CAD build for the part. Positions are in the model's coordinates, mm. Round coordinates to 2 decimals unless told otherwise and drop trailing zeros. Loops run counter-clockwise (first coordinate to the right, second up) from the corner with the lowest first, then second, coordinate; pieces in that order, holes last. Notation, with made-up numbers: M 53,26 L 87,26 A7 cw 87,33 Z; hole C 78.5,10 d8. An arc over 180 degrees is marked long. Use one line per item in the form item = value.
from build123d import *

# Parameters (mm, degrees)
F2_W     = 25.146
F2_H     = 4.7498
F3_DEPTH = 34.6974
F4_R     = 0.381


with BuildPart() as f1:
    # F0 (on Right) → F1 (revolve)
    with BuildSketch(Plane.YZ):
        Polygon((-12.6492, 0.1524), (-12.6492, 34.6964), (-16.6624, 34.6964), (-16.6624, 31.6484), (-13.8938, 31.6484), (-13.8938, 12.8524), (-13.2842, 0.1524), align=None)
    revolve(axis=Axis((0, 0, 4.6482), (0, 0, -1)))

    # F2 (on Top) → F3 (cut, through all)
    with BuildSketch(Plane.XY):
        with Locations((-12.827, 0)):
            Rectangle(F2_W, F2_H)
    extrude(amount=F3_DEPTH, mode=Mode.SUBTRACT)

    # F4
    f4_edges = [f1.edges().sort_by_distance(p)[0] for p in [
        (-13.379864, -2.3749, 6.502395),
        (-13.689322, -2.3749, 22.2504),
        (-13.379864, 2.3749, 6.502395),
        (-13.689322, 2.3749, 22.2504),
        (-15.090803, -2.3749, 31.6484),
        (-15.090803, 2.3749, 31.6484),
        (12.6492, 0, 34.6964),
        (13.8938, 0, 12.8524),
    ]]
    fillet(f4_edges, radius=F4_R)


solid = f1.part
1. Probe line 1 along Y through (x, z) = (0, 15); line 2 along Y through (x, z) = (3.5, 6); line 3 along X through (y, z) = (10.5, 4). List the from-to ranges inside material, lowest first. Write a range as from..to.
Completed:
line_1 = -13.89..-12.65, 12.65..13.89
line_2 = -13.11..-12.16, 12.16..13.11
line_3 = -8.44..-7.05, 7.05..8.44
2. Cut at C-C on z = 13.5. Write the cut outline in (x, y), and give its area (3 significant figures).
Completed:
outline = M -13.6,-2.83 A13.89 ccw long -13.6,2.83 A0.38 ccw -13.23,2.37 L -12.42,2.37 A12.65 cw long -12.42,-2.37 L -13.23,-2.37 A0.38 ccw Z
area = 97.7 mm2
3. Cut at B-B on y = 0. Write the cut outline in (x, z), and give its area (3 significant figures).
Completed:
outline = M 12.65,0.15 L 13.28,0.15 L 13.89,12.85 L 13.89,31.65 L 16.66,31.65 L 16.66,34.7 L 13.03,34.7 A0.38 ccw 12.65,34.32 Z
area = 47.5 mm2
4. Pull direction Y, two halves, no side cores. Call faces 1 (the face through (-13, 2.375, 22)), 2 (the face through (13.882, 0.571, 22.119)), 3 (the face through (-13, -2.375, 22)), 4 (the face through (14, 4, 31.648)): +Y half, -Y half, draft (parallel to the pull), parting line (faces both ways), or undercut.
Completed:
face_1 = undercut
face_2 = parting line
face_3 = undercut
face_4 = draft
5. Cut at A-A on x = 0. Write the cut outline in (y, z).
Completed:
outline = M -16.66,31.65 L -13.89,31.65 L -13.89,12.85 L -13.28,0.15 L -12.65,0.15 L -12.65,34.32 A0.38 ccw -13.03,34.7 L -16.66,34.7 Z; M 12.65,0.15 L 13.28,0.15 L 13.89,12.85 L 13.89,31.65 L 16.66,31.65 L 16.66,34.7 L 13.03,34.7 A0.38 ccw 12.65,34.32 Z
6. Drop flat-ended pins along their axis: P1, Ø12, axis at y = 12, z = 24.5, coming from the +X side; P2, Ø12, axis at y = -9.5, z = 18.5, coming from the +X side; P3, Ø8, axis at y = -3, z = 5, coming from the +X side; P4, Ø8, axis at x = -0.5, y = -7, coming from the +Z side. Give the stop position or say it passes through.
Completed:
P1 = 12.53
P2 = 13.45
P3 = 13.66
P4 = through
